Check sheet for the modelled part. Datum: model origin and axes. Units: mm. Round coordinates to 2 decimals unless told otherwise and drop trailing zeros. Answer in a Markdown table with one row per item.
```python
from build123d import *

# Parameters (mm, degrees)
SKETCH1_W           = 205.16159644
SKETCH1_H           = 139.144251052
BOSS_EXTRUDE1_DEPTH = 2.54
SKETCH3_R           = 1.9304
CUT_EXTRUDE1_DEPTH  = 124.973998942


with BuildPart() as part:
    # Sketch1 → Boss-Extrude1 (new body)
    with BuildSketch(Plane(origin=(0, 0, 0), x_dir=(1, 0, 0), z_dir=(0, 1, 0))):
        Rectangle(SKETCH1_W, SKETCH1_H)
    extrude(amount=BOSS_EXTRUDE1_DEPTH)

    # Sketch3 → Cut-Extrude1 (cut, through all)
    with BuildSketch(Plane(origin=(0, 2.54, 0), x_dir=(1, 0, 0), z_dir=(0, 1, 0))):
        with Locations(Location((-81.293768085, 36.19177457, 0), (0, 0, 270))):
            Circle(SKETCH3_R)
        with Locations(Location((-56.300168085, 36.19177457, 0), (0, 0, 270))):
            Circle(SKETCH3_R)
        with Locations(Location((-42.832492591, 36.19177457, 0), (0, 0, 270))):
            Circle(SKETCH3_R)
        with Locations(Location((-17.838892591, 36.19177457, 0), (0, 0, 270))):
            Circle(SKETCH3_R)
        with Locations(Location((-0.229233582, 35.924108913, 0), (0, 0, 270))):
            Circle(SKETCH3_R)
        with Locations(Location((24.764366418, 35.924108913, 0), (0, 0, 270))):
            Circle(SKETCH3_R)
        with Locations(Location((46.220152976, 35.873923159, 0), (0, 0, 270))):
            Circle(SKETCH3_R)
        with Locations(Location((71.213752976, 35.873923159, 0), (0, 0, 270))):
            Circle(SKETCH3_R)
        with BuildLine():
            Line((-62.535868085, 40.90347457), (-75.058068085, 40.90347457))
            ThreePointArc((-75.058068085, 40.90347457), (-76.969282019, 40.096622494), (-77.724090306, 38.164262946))
            Line((-77.724090306, 38.164262946), (-76.934091112, 33.68395488))
            ThreePointArc((-76.934091112, 33.68395488), (-76.02192339, 32.10403404), (-74.307608835, 31.48007457))
            Line((-74.307608835, 31.48007457), (-63.286327336, 31.48007457))
            ThreePointArc((-63.286327336, 31.48007457), (-61.572012781, 32.10403404), (-60.659845059, 33.68395488))
            Line((-60.659845059, 33.68395488), (-59.869845865, 38.164262946))
            ThreePointArc((-59.869845865, 38.164262946), (-60.624654152, 40.096622494), (-62.535868085, 40.90347457))
        make_face()
        with BuildLine():
            Line((-24.074592591, 40.90347457), (-36.596792591, 40.90347457))
            ThreePointArc((-36.596792591, 40.90347457), (-38.508006525, 40.096622494), (-39.262814812, 38.164262946))
            Line((-39.262814812, 38.164262946), (-38.472815618, 33.68395488))
            ThreePointArc((-38.472815618, 33.68395488), (-37.560647896, 32.10403404), (-35.846333341, 31.48007457))
            Line((-35.846333341, 31.48007457), (-24.825051842, 31.48007457))
            ThreePointArc((-24.825051842, 31.48007457), (-23.110737287, 32.10403404), (-22.198569565, 33.68395488))
            Line((-22.198569565, 33.68395488), (-21.408570371, 38.164262946))
            ThreePointArc((-21.408570371, 38.164262946), (-22.163378658, 40.096622494), (-24.074592591, 40.90347457))
        make_face()
        with BuildLine():
            Line((18.528666418, 40.635808913), (6.006466418, 40.635808913))
            ThreePointArc((6.006466418, 40.635808913), (4.095252484, 39.828956838), (3.340444197, 37.89659729))
            Line((3.340444197, 37.89659729), (4.130443391, 33.416289223))
            ThreePointArc((4.130443391, 33.416289223), (5.042611113, 31.836368383), (6.756925668, 31.212408913))
            Line((6.756925668, 31.212408913), (17.778207167, 31.212408913))
            ThreePointArc((17.778207167, 31.212408913), (19.492521722, 31.836368383), (20.404689444, 33.416289223))
            Line((20.404689444, 33.416289223), (21.194688638, 37.89659729))
            ThreePointArc((21.194688638, 37.89659729), (20.439880351, 39.828956838), (18.528666418, 40.635808913))
        make_face()
        with BuildLine():
            Line((64.978052976, 40.585623159), (52.455852976, 40.585623159))
            ThreePointArc((52.455852976, 40.585623159), (50.544639042, 39.778771083), (49.789830755, 37.846411536))
            Line((49.789830755, 37.846411536), (50.579829949, 33.366103469))
            ThreePointArc((50.579829949, 33.366103469), (51.491997671, 31.786182629), (53.206312227, 31.162223159))
            Line((53.206312227, 31.162223159), (64.227593725, 31.162223159))
            ThreePointArc((64.227593725, 31.162223159), (65.94190828, 31.786182629), (66.854076003, 33.366103469))
            Line((66.854076003, 33.366103469), (67.644075197, 37.846411536))
            ThreePointArc((67.644075197, 37.846411536), (66.88926691, 39.778771083), (64.978052976, 40.585623159))
        make_face()
    extrude(amount=-CUT_EXTRUDE1_DEPTH, mode=Mode.SUBTRACT)


solid = part.part
```
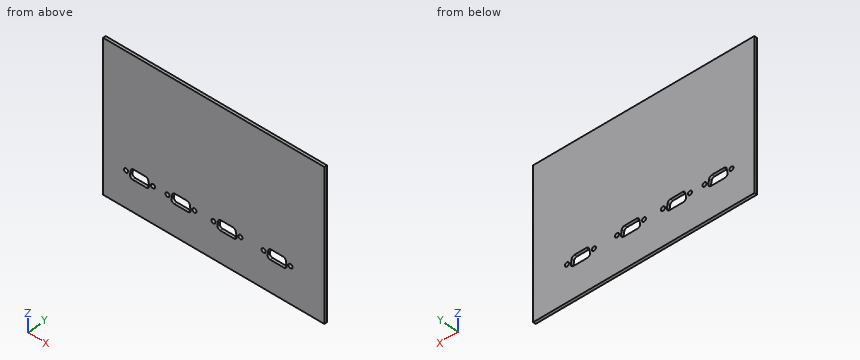
1. Scan lines: L1, parallel to X at y = 0.85, z = -33.5; L2, parallel to X at y = 2.4, z = -39; L3, parallel to Z at x = 9.5, y = 2.2. Record each from-to range of solid material in increasing order.
Found:
| item | result |
|---|---|
| L1 | x = -102.58 to -76.89, -60.7 to -38.43, -22.24 to 4.12, 20.42 to 50.56, 66.88 to 102.58 |
| L2 | x = -102.58 to -77.61, -59.98 to -39.15, -21.52 to 3.55, 20.99 to 50.02, 67.42 to 102.58 |
| L3 | z = -69.57 to -40.64, -31.21 to 69.57 |
2. Go/stop test with a flat-tipped pin: pin 1 (3.5 mm diameter, centred on x = 24.76, z = -35.92, fed in from -Y). Record where the tip stops, or that it passes through.
Found:
| item | result |
|---|---|
| pin 1 | passes through |
3. Section check A-A, the plane y = 0.6. Count the separate pieces of the cut face and the enclosed holes in it, and give its area (3 significant figures).
Found:
| item | result |
|---|---|
| separate pieces | 1 |
| enclosed holes | 12 |
| area | 27,800 mm2 |
